Source: CAD feature listing. Evaluate the final solid. Frame: model axes, mm. Give positions to 0.01 mm unless a question says otherwise; leave off trailing zeros. Loops run counter-clockwise (first coordinate to the right, second up) from the corner with the lowest first, then second, coordinate; pieces in that order, holes last. Notation, with made-up numbers: M -39,62 L -13,62 A15 ccw -13,67 Z; hole C -23.75,-29 d4. An arc over 180 degrees is marked long. Answer in a Markdown table with one row per item.
```python
from build123d import *

# Parameters (mm, degrees)
ESBO_O1_R                = 2
RESSALTO_EXTRUS_O1_DEPTH = 0.5


with BuildPart() as part:
    # Esboço1 → Ressalto-extrusão1 (new body)
    # profile 1 of 2: a face of its own
    with BuildSketch(Plane.XY):
        Polygon((210, -50), (210, 0), (52.5, 0), (52.5, -75), (105, -75), align=None)
        with Locations((57.5, -70)):
            Circle(ESBO_O1_R, mode=Mode.SUBTRACT)
        with Locations((205, -46.050706394)):
            Circle(ESBO_O1_R, mode=Mode.SUBTRACT)
    # profile 2 of 2: a face of its own
    with BuildSketch(Plane.XY):
        Polygon((210, 0), (210, 50), (105, 75), (52.5, 75), (52.5, 0), align=None)
        with Locations((57.5, 70)):
            Circle(ESBO_O1_R, mode=Mode.SUBTRACT)
        with Locations((205, 46.050706394)):
            Circle(ESBO_O1_R, mode=Mode.SUBTRACT)
    extrude(amount=RESSALTO_EXTRUS_O1_DEPTH)


solid = part.part
```
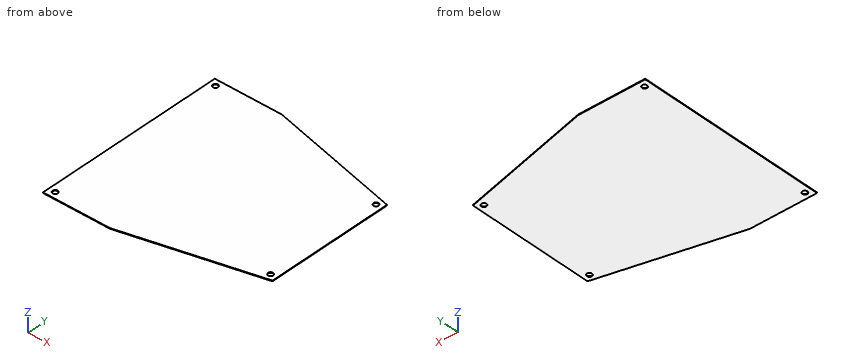
Q1. Section query A-A (x = 57.5). Output: boundary loops of the cut face in (y, z).
Values follow:
| item | result |
|---|---|
| outline | M -75,0 L -72,0 L -72,0.5 L -75,0.5 Z; M -68,0 L 68,0 L 68,0.5 L -68,0.5 Z; M 72,0 L 75,0 L 75,0.5 L 72,0.5 Z |
Q2. Section query C-C (z = 0.4). Output: boundary loops of the cut face in (x, y).
Values follow:
| item | result |
|---|---|
| outline | M 52.5,-75 L 105,-75 L 210,-50 L 210,50 L 105,75 L 52.5,75 Z; hole C 57.5,-70 d4; hole C 57.5,70 d4; hole C 205,-46.05 d4; hole C 205,46.05 d4 |
Q3. Ray query, probe 1 along Y at (x, z) = (57.5, 0.45); probe 2 along Y at (x, z) = (205, 0.3); probe 3 along Y at (x, z) = (185, 0.4). Return the intervals inside material, ascending. Write a range as from..to.
Values follow:
| item | result |
|---|---|
| probe 1 | -75..-72, -68..68, 72..75 |
| probe 2 | -51.19..-48.05, -44.05..44.05, 48.05..51.19 |
| probe 3 | -55.95..55.95 |
Q4. Section query D-D (x = 205). Output: boundary loops of the cut face in (y, z).
Values follow:
| item | result |
|---|---|
| outline | M -51.19,0 L -48.05,0 L -48.05,0.5 L -51.19,0.5 Z; M -44.05,0 L 44.05,0 L 44.05,0.5 L -44.05,0.5 Z; M 48.05,0 L 51.19,0 L 51.19,0.5 L 48.05,0.5 Z |
Q5. Contact query for a flat-ended pin moving along its axis: pin 1 Ø2.5 at (x, y) = (205, -46.05) entering from +Z. Output: stop coordinate, or through.
Values follow:
| item | result |
|---|---|
| pin 1 | through |
Q6. Section query B-B (y = 70). Output: boundary loops of the cut face in (x, z), plus the area to 4 significant figures.
Values follow:
| item | result |
|---|---|
| outline | M 52.5,0 L 55.5,0 L 55.5,0.5 L 52.5,0.5 Z; M 59.5,0 L 126,0 L 126,0.5 L 59.5,0.5 Z |
| area | 34.75 mm^2 |
